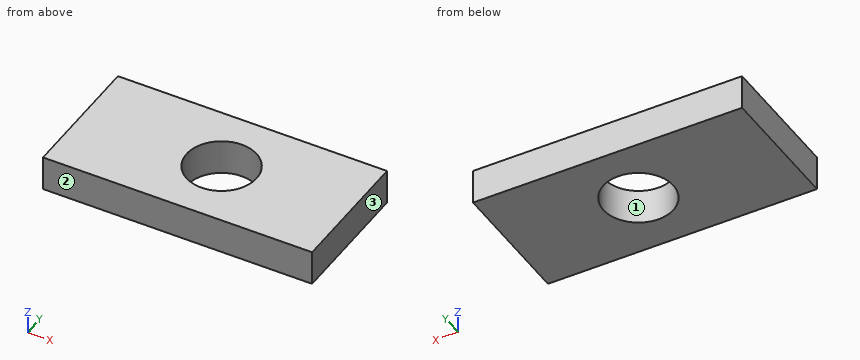
from build123d import *

# Parameters (mm, degrees)
SKETCH_W  = 230.942398
SKETCH_H  = 112.814285
SKETCH_R  = 30
PAD_DEPTH = 30


with BuildPart() as part:
    # Sketch → Pad (new body)
    with BuildSketch(Plane.XY):
        with Locations((-5.425507, -0.407142)):
            Rectangle(SKETCH_W, SKETCH_H)
        Circle(SKETCH_R, mode=Mode.SUBTRACT)
    extrude(amount=PAD_DEPTH)


solid = part.part
Can you work these out from the model? Positions are in its coordinate system, mm. Face numbers are marked on the shaded views. Coordinates: 2 decimals unless noted, no trailing zeros. Write each loop counter-clockwise with the first axis right and the second up, starting at its lowest first coordinate (ties: lowest second). Pieces come first, ordered by that corner, then holes. Notation, with made-up numbers: (17, -27.5) - (52, -27.5) arc R24 ccw to (52, -16.5) - close; hole circle Ø5 at (84.5, 41.5). An arc over 180 degrees is marked (long way). Return JSON: item names as keys, results as strings. Group by question number.
Item 1: We'd pull the mould along X, two halves only. Please class the marked faces 1, 2 and 3: pulls with the +X half, pulls with the -X half, needs draft (parallel to the pull), parting line crosses it, or undercut.
Item 2: If we section it at C-C (z = 17.75): Write out the boundary of the cut face in (x, y).
Item 3: Please list where these lines run through material, in increasing order: probe 1 along Y at (x, z) = (0, 7.25); probe 2 along Y at (x, z) = (4.5, 16.25); probe 3 along X at (y, z) = (-2, 16.75).
Item 4: If we section it at B-B (y = 0): Write out the boundary of the cut face in (x, z).
Item 5: If we section it at A-A (x = 0): Write out the boundary of the cut face in (y, z).
Return value:
{
 "1": {"face 1": "undercut", "face 2": "needs draft", "face 3": "pulls with the +X half"},
 "2": {"outline": "(-120.9, -56.81) - (110.05, -56.81) - (110.05, 56) - (-120.9, 56) - close; hole circle Ø60 at (0, 0)"},
 "3": {"probe 1": "y = -56.81 to -30, 30 to 56", "probe 2": "y = -56.81 to -29.66, 29.66 to 56", "probe 3": "x = -120.9 to -29.93, 29.93 to 110.05"},
 "4": {"outline": "(-120.9, 0) - (-30, 0) - (-30, 30) - (-120.9, 30) - close; (30, 0) - (110.05, 0) - (110.05, 30) - (30, 30) - close"},
 "5": {"outline": "(-56.81, 0) - (-30, 0) - (-30, 30) - (-56.81, 30) - close; (30, 0) - (56, 0) - (56, 30) - (30, 30) - close"}
}
